Build history of the part. All positions in model axes, mm. Face numbers are marked on the shaded views. A direction names the side the tool comes from. Give positions to 0.01 mm unless a question says otherwise; leave off trailing zeros. Loops run counter-clockwise (first coordinate to the right, second up) from the corner with the lowest first, then second, coordinate; pieces in that order, holes last. Notation, with made-up numbers: (-12, 69) -> (40, 69) arc R17 cw to (40, 96) -> close; hole circle Ø7 at (-29, -12). An arc over 180 degrees is marked (long way). Answer as a JSON object with one key per item and string values. Group by question number.
Q1. Drop flat-ended pins along their axis: pin 1 (4 mm diameter, centred on y = 15.5, z = 5.5, fed in from -X); pin 2 (1.5 mm diameter, centred on x = -6.5, z = 3.5, fed in from -Y); pin 3 (1 mm diameter, centred on y = -41, z = 2, fed in from -X). Give the stop position or say it passes through.
Q2. Wall check: probe 1 along X at (y, z) = (0, 4); probe 2 along Y at (x, z) = (0, 9); probe 3 along X at (y, z) = (-7.5, 5). Give the ranges that are in metal, low to high. Write a range as from..to.
Q3. Band-saw the part on D-D, the plane y = -29. Write the cut outline in (x, z), plus the area to 3 significant figures.
Q4. Band-saw the part on C-C, the plane x = -63. Write the cut outline in (y, z).
Q5. Band-saw the part on B-B, the plane z = 5.5. Count the separate pieces of the cut face and the enclosed holes in it, plus the area to 3 significant figures.
Q6. Two-plate mould, pull along Y, no slides. Class the marked faces 1, 2 and 3: pulls with the +Y half, pulls with the -Y half, needs draft (parallel to the pull), parting line crosses it, or undercut.
Q7. Tool access for the marked faces 4 and 5: list every direction of +Z, -Z, +X, -X, +Y, -Y with a clear straight run to the whole face (end or side of a thin tool).
Q8. Band-saw the part on A-A, the plane y = 0. Write the cut outline in (x, z).
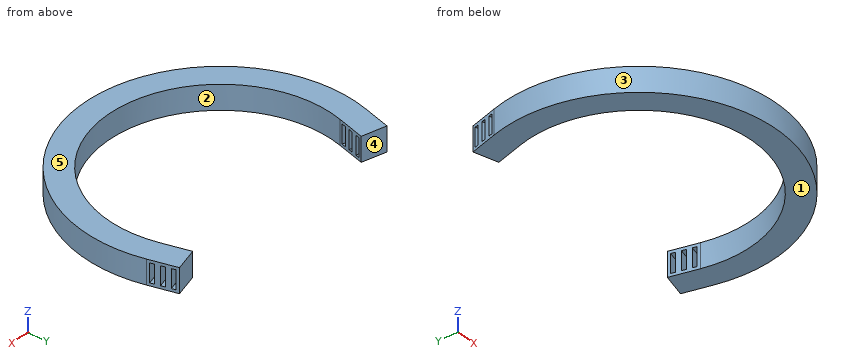
from build123d import *

# Parameters (mm, degrees)
F1_DEPTH = 13
F2_W     = 2.2
F2_H     = 3.9
F3_DEPTH = 25
F4_W     = 2.2
F4_H     = 10
F5_DEPTH = 25


with BuildPart() as f1:
    # F0 (on Top) → F1 (new body)
    with BuildSketch(Plane.XY):
        with BuildLine():
            ThreePointArc((57.95555, 15.529143), (0, -60), (-57.95555, 15.529143))
            Line((-57.95555, 15.529143), (-54.073264, 30.01803))
            Line((-54.073264, 30.01803), (-66.6303, 33.382678))
            Line((-66.6303, 33.382678), (-70.512585, 18.89379))
            ThreePointArc((-70.512585, 18.89379), (0, -73), (70.512585, 18.89379))
            Line((70.512585, 18.89379), (66.6303, 33.382678))
            Line((66.6303, 33.382678), (54.073264, 30.01803))
            Line((54.073264, 30.01803), (57.95555, 15.529143))
        make_face()
    extrude(amount=F1_DEPTH)

    # F2 (on face) → F3 (cut)
    with BuildSketch(Plane(origin=(70.512585, 18.89379, 0), x_dir=(-0.258819, 0.965926, 0), z_dir=(0.965926, 0.258819, 0))):
        Polygon((1.5, 11.5), (1.5, 7.6), (1.5, 1.5), (3.7, 1.5), (3.7, 7.6), (3.7, 11.5), align=None)
        Polygon((8.6, 11.5), (6.4, 11.5), (6.4, 7.6), (6.4, 1.5), (8.6, 1.5), (8.6, 7.6), align=None)
        Polygon((13.5, 11.5), (11.3, 11.5), (11.3, 7.6), (11.3, 1.5), (13.5, 1.5), (13.5, 7.6), align=None)
        with Locations((542.279418, 3.45)):
            Rectangle(F2_W, F2_H)
    extrude(amount=-F3_DEPTH, mode=Mode.SUBTRACT)

    # F4 (on face) → F5 (cut)
    with BuildSketch(Plane(origin=(-70.512585, 18.89379, 0), x_dir=(-0.258819, -0.965926, 0), z_dir=(-0.965926, 0.258819, 0))):
        with Locations((-2.6, 6.5)):
            Rectangle(F4_W, F4_H)
        with Locations((-7.5, 6.5)):
            Rectangle(F4_W, F4_H)
        with Locations((-12.4, 6.5)):
            Rectangle(F4_W, F4_H)
    extrude(amount=-F5_DEPTH, mode=Mode.SUBTRACT)


solid = f1.part
Worked answers:
{
 "1": {"pin 1": "x = -71.74", "pin 2": "y = -72.77", "pin 3": "x = -60.74"},
 "2": {"probe 1": "-73..-60, 60..73", "probe 2": "-73..-60", "probe 3": "-72.61..-59.53, 59.53..72.61"},
 "3": {"outline": "(-66.99, 0) -> (-52.53, 0) -> (-52.53, 13) -> (-66.99, 13) -> close; (52.53, 0) -> (66.99, 0) -> (66.99, 13) -> (52.53, 13) -> close", "area": "376 mm2"},
 "4": {"outline": "(-36.88, 0) -> (32.41, 0) -> (32.41, 13) -> (-36.88, 13) -> close; hole (18.43, 1.5) -> (20.71, 1.5) -> (20.71, 11.5) -> (18.43, 11.5) -> close; hole (23.51, 1.5) -> (25.78, 1.5) -> (25.78, 11.5) -> (23.51, 11.5) -> close; hole (28.58, 1.5) -> (30.86, 1.5) -> (30.86, 11.5) -> (28.58, 11.5) -> close"},
 "5": {"separate pieces": "7", "enclosed holes": "0", "area": "3,390 mm2"},
 "6": {"face 1": "needs draft", "face 2": "undercut", "face 3": "parting line crosses it"},
 "7": {"face 4": "+Z, -Z, +Y", "face 5": "+Z, +X, -X, +Y, -Y"},
 "8": {"outline": "(-73, 0) -> (-60, 0) -> (-60, 13) -> (-73, 13) -> close; (60, 0) -> (73, 0) -> (73, 13) -> (60, 13) -> close"}
}
